Design review of the part built by this model. Coordinates are the model's own, in mm. A direction names the side the tool comes from. Coordinates: 2 decimals unless noted, no trailing zeros. Write item = value, one per line.
```python
from build123d import *

# Parameters (mm, degrees)
F0_W     = 50.8
F0_H     = 19.05
F1_DEPTH = 927.1
F2_W     = 122.43557321
F2_H     = 50.8
F2_W_2   = 343.1604206562
F2_W_3   = 264.5317912102
F3_DEPTH = 25.4
F4_R     = 0.79375
F5_DEPTH = 25.4
F6_R     = 4.7625
F7_DEPTH = 25.4


# Not quite as in the source:
# - a feature names something its author has since deleted; it is built from what else it names


with BuildPart() as f1:
    # F0 (on Top) → F1 (new body)
    with BuildSketch(Plane.XY):
        Rectangle(F0_W, F0_H)
    extrude(amount=F1_DEPTH)

    # F2 (on Front) → F3 (cut)
    with BuildSketch(Plane.XZ):
        with Locations((22.4465244144, 177.8)):
            Rectangle(F2_W, F2_H)
        with Locations((-38.7818217278, 901.7)):
            Rectangle(F2_W_2, F2_H)
        with Locations((-47.6498156786, 514.35)):
            Rectangle(F2_W_3, F2_H)
    extrude(amount=F3_DEPTH, mode=Mode.SUBTRACT)

    # F4 (on Front) → F5 (cut)
    with BuildSketch(Plane.XZ):
        with Locations((9.525, 254)):
            Circle(F4_R)
        with Locations((9.525, 307.975)):
            Circle(F4_R)
        with Locations((9.525, 771.525)):
            Circle(F4_R)
        with Locations((9.525, 825.5)):
            Circle(F4_R)
        with Locations((-9.525, 771.525)):
            Circle(F4_R)
        with Locations((-9.525, 825.5)):
            Circle(F4_R)
        with Locations((-9.525, 254)):
            Circle(F4_R)
        with Locations((-9.525, 307.975)):
            Circle(F4_R)
    extrude(amount=-F5_DEPTH, mode=Mode.SUBTRACT)

    # F6 (on Front) → F7 (cut)
    with BuildSketch(Plane.XZ):
        with Locations((0, 247.65)):
            Circle(F6_R)
    extrude(amount=F7_DEPTH, mode=Mode.SUBTRACT)


solid = f1.part
```
Q1. Wall thickness on line 1 (X direction, y = 2.5, z = 254); line 2 (Z direction, x = -12, y = -1.75); line 3 (Z direction, x = 9.5, y = 6.5): over which ranges is each line inside the solid? List them lowest first.
Check result:
line_1 = -25.4 to -10.32, -8.73 to 8.73, 10.32 to 25.4
line_2 = 0 to 152.4, 203.2 to 488.95, 539.75 to 876.3
line_3 = 0 to 253.21, 254.79 to 307.18, 308.77 to 770.73, 772.32 to 824.71, 826.29 to 927.1
Q2. Machinability: for faces 1 (the flat face through (25.4, 0, 457)), 2 (the flat face through (0, 0, 902)), 3 (the flat face through (0, 0, 178)), which of the approach directions +Z, -Z, +X, -X, +Y, -Y give a long, thin tool a straight path to every point of the face, cutting with its end or side? Answer none if there is none.
Check result:
face_1 = +Z, -Z, +X, +Y, -Y
face_2 = +Z, +X, -X, -Y
face_3 = +X, -X, -Y
Q3. For P1, Ø1.3, axis at x = -9.5, z = 825.5, coming from the +Y side; P2, Ø7.5, axis at x = -7, y = -6, coming from the +Z side; P3, Ø5, axis at x = -0.5, z = 246.5, coming from the -Y side, all flat-tipped, find the tip position at first contact; note any pin that passes through.
Check result:
P1 = 0
P2 = 876.3
P3 = 0
